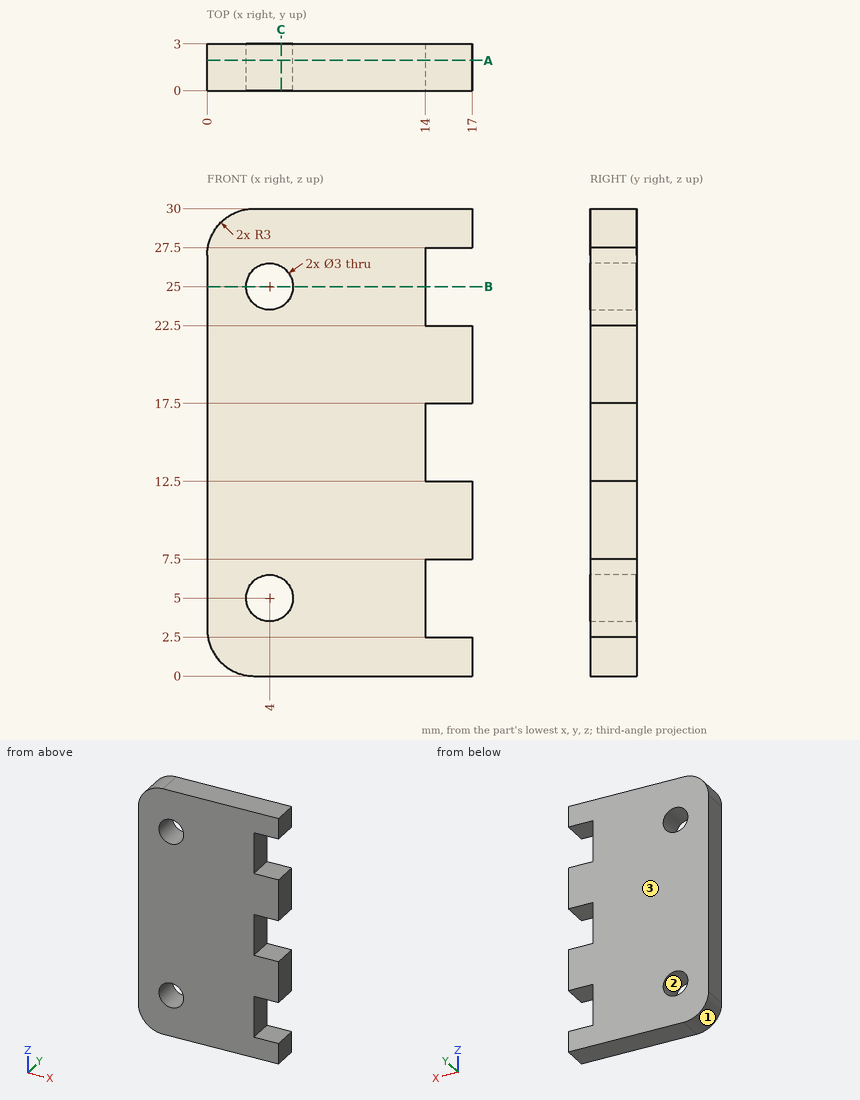
Could you check a few things on this drawing? It's one solid part, dimensions in mm from its lowest x, y, z. Coordinates: 2 decimals unless noted, no trailing zeros. Order: outer loops, then holes, each group sorted by start corner. A loop starts at its lowest first (then second) coordinate and runs counter-clockwise, first axis right, second up.
1. If we section it at B-B (z = 25): Please give me the cut outline in (x, y), then the cut area to 3 significant figures.
2. Thinking about a two-plate mould opening in Z: for the marked faces 1, 2 and 3, which applies, +Z half, -Z half, draft (parallel to the pull), parting line (faces both ways), or undercut?
3. I need wall thicknesses on line 1 (Z direction, x = 14.5, y = 2.8); line 2 (X direction, y = 1.4, z = 25); line 3 (X direction, y = 2.75, z = 24.5). Which ranges of each line are inside material? Lowest first, please.
4. If we section it at C-C (x = 4.75): Please give me the cut outline in (y, z), then the cut area to 3 significant figures.
5. If we section it at A-A (y = 1.95): Please give me the cut outline in (x, z).
6. I'm going to push a flat-ended pin straight in: pin 1 (1.5 mm diameter, centred on x = 5, z = 4, fed in from +Y). Where does the tip first touch, or does it pass through?
Entries:
1. outline: (0, 0) - (2.5, 0) - (2.5, 3) - (0, 3) - close; (5.5, 0) - (14, 0) - (14, 3) - (5.5, 3) - close
1. area: 33.0 mm2
2. face 1: -Z half
2. face 2: undercut
2. face 3: draft
3. line 1: z = 0 to 2.5, 7.5 to 12.5, 17.5 to 22.5, 27.5 to 30
3. line 2: x = 0 to 2.5, 5.5 to 14
3. line 3: x = 0 to 2.59, 5.41 to 14
4. outline: (0, 0) - (3, 0) - (3, 3.7) - (0, 3.7) - close; (0, 6.3) - (3, 6.3) - (3, 23.7) - (0, 23.7) - close; (0, 26.3) - (3, 26.3) - (3, 30) - (0, 30) - close
4. area: 74.4 mm2
5. outline: (0, 3) arc R3 ccw to (3, 0) - (17, 0) - (17, 2.5) - (14, 2.5) - (14, 7.5) - (17, 7.5) - (17, 12.5) - (14, 12.5) - (14, 17.5) - (17, 17.5) - (17, 22.5) - (14, 22.5) - (14, 27.5) - (17, 27.5) - (17, 30) - (3, 30) arc R3 ccw to (0, 27) - close; hole circle Ø3 at (4, 5); hole circle Ø3 at (4, 25)
6. pin 1: stops at y = 3
